Answer from the drawing. Dimensions are ordinates in mm from the lowest x, y and z of the part. Round coordinates to 2 decimals unless told otherwise and drop trailing zeros. Write each loop counter-clockwise with the first axis right and the second up, starting at its lowest first coordinate (ties: lowest second). Pieces come first, ordered by that corner, then holes. Notation, with made-up numbers: (-33, 62.25) - (4, 62.25) arc R28 ccw to (4, 101.25) - close; hole circle Ø10 at (-3.5, -8). An arc over 180 degrees is marked (long way). Answer as a JSON object with one key per item and string values.
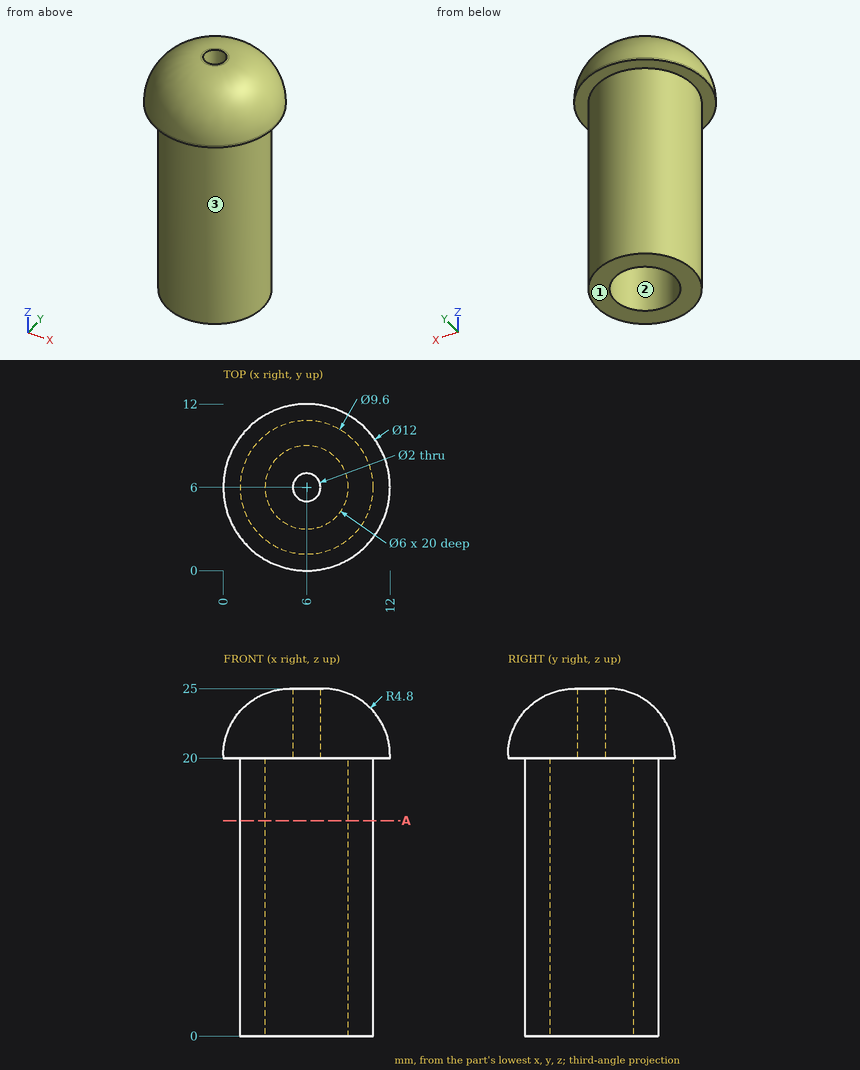
Item 1: Each of these flat-tipped pins is pushed along its axis until it touches: P1, Ø3, axis at x = 2, z = 7.5, coming from the +Y side; P2, Ø1, axis at x = 10.5, y = 6.5, coming from the +Z side; P3, Ø3, axis at y = 7, z = 9.5, coming from the -X side. Where does it stop, or does it pass through?
Results found:
{"P1": "y = 10.1", "P2": "z = 24.08", "P3": "x = 1.2"}
Item 2: A cutting plane is placed at A-A (z = 15.5). Write down the section's boundary in (x, y).
Results found:
{"outline": "circle Ø9.6 at (6, 6); hole circle Ø6 at (6, 6)"}
Item 3: Consider line 1 along Y through (x, z) = (6, 10.5); line 2 along X through (y, z) = (8.75, 16.5); line 3 along X through (y, z) = (6.5, 4.25). Determine where each line is inside the solid, lowest interval first.
Results found:
{"line 1": "1.2 to 3, 9 to 10.8", "line 2": "2.07 to 4.8, 7.2 to 9.93", "line 3": "1.23 to 3.04, 8.96 to 10.77"}
Item 4: Determine the mould class of the marked faces 1, 2 and 3 for opening direction Y: pulls with the +Y half, pulls with the -Y half, needs draft (parallel to the pull), parting line crosses it, or undercut.
Results found:
{"face 1": "needs draft", "face 2": "undercut", "face 3": "parting line crosses it"}
